Part model, mm, in its own coordinate system. Round coordinates to 2 decimals unless told otherwise and drop trailing zeros. Write each loop counter-clockwise with the first axis right and the second up, starting at its lowest first coordinate (ties: lowest second). Pieces come first, ordered by that corner, then holes.
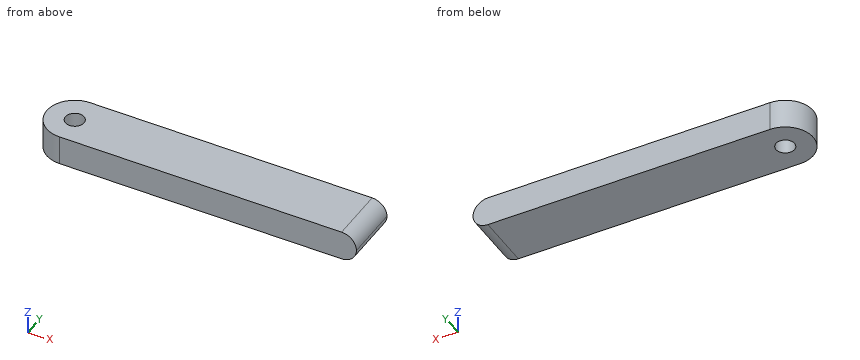
```python
from build123d import *

# Parameters (mm, degrees)
ESQUISSE1_R        = 2.5
BOSS_EXTRU_1_DEPTH = 8
CONG_1_R           = 4


with BuildPart() as part:
    # Esquisse1 → Boss.-Extru.1 (new body)
    with BuildSketch(Plane.XY):
        with BuildLine():
            Line((0, 7.5), (80, 7.5))
            Line((80, 7.5), (80, -7.5))
            Line((80, -7.5), (0, -7.5))
            ThreePointArc((0, -7.5), (-7.5, 0), (0, 7.5))
        make_face()
        Circle(ESQUISSE1_R, mode=Mode.SUBTRACT)
    extrude(amount=BOSS_EXTRU_1_DEPTH)

    # Congé1
    cong_1_edges = [part.edges().sort_by_distance(p)[0] for p in [
        (80, 0, 0),
        (80, 0, 8),
    ]]
    fillet(cong_1_edges, radius=CONG_1_R - 0.0001)  # a hair under: the kernel refuses the full size


solid = part.part
```
Q1. Cut at B-B on z = 5.5. Write the cut outline in (x, y).
Values follow:
outline: (0, -7.5) - (79.71, -7.5) - (79.71, 7.5) - (0, 7.5) arc R7.5 ccw to start; hole circle Ø5 at (0, 0)
Q2. Wall check: L1, parallel to Y at x = 0, z = 2.75; L2, parallel to X at y = -0.5, z = 4.5; L3, parallel to X at y = -4.5, z = 1.5. Give the ranges that are in metal, low to high.
Values follow:
L1: y = -7.5 to -2.5, 2.5 to 7.5
L2: x = -7.48 to -2.45, 2.45 to 79.97
L3: x = -6 to 79.12
Q3. Cut at D-D on z = 0.75. Write the cut outline in (x, y).
Values follow:
outline: (0, -7.5) - (78.33, -7.5) - (78.33, 7.5) - (0, 7.5) arc R7.5 ccw to start; hole circle Ø5 at (0, 0)
